Source: three-view drawing plus pictorial views. Frame: mm from the lowest corner of the part. Coordinates: 2 decimals unless noted, no trailing zeros. Write each loop counter-clockwise with the first axis right and the second up, starting at its lowest first coordinate (ties: lowest second). Pieces come first, ordered by that corner, then holes. Notation, with made-up numbers: (-12, 15) -> (13, 15) arc R13 ccw to (13, 22) -> close; hole circle Ø7 at (67, 64.5). An arc over 180 degrees is marked (long way). One line per question, with ' | ' between items. Start each with the question number.
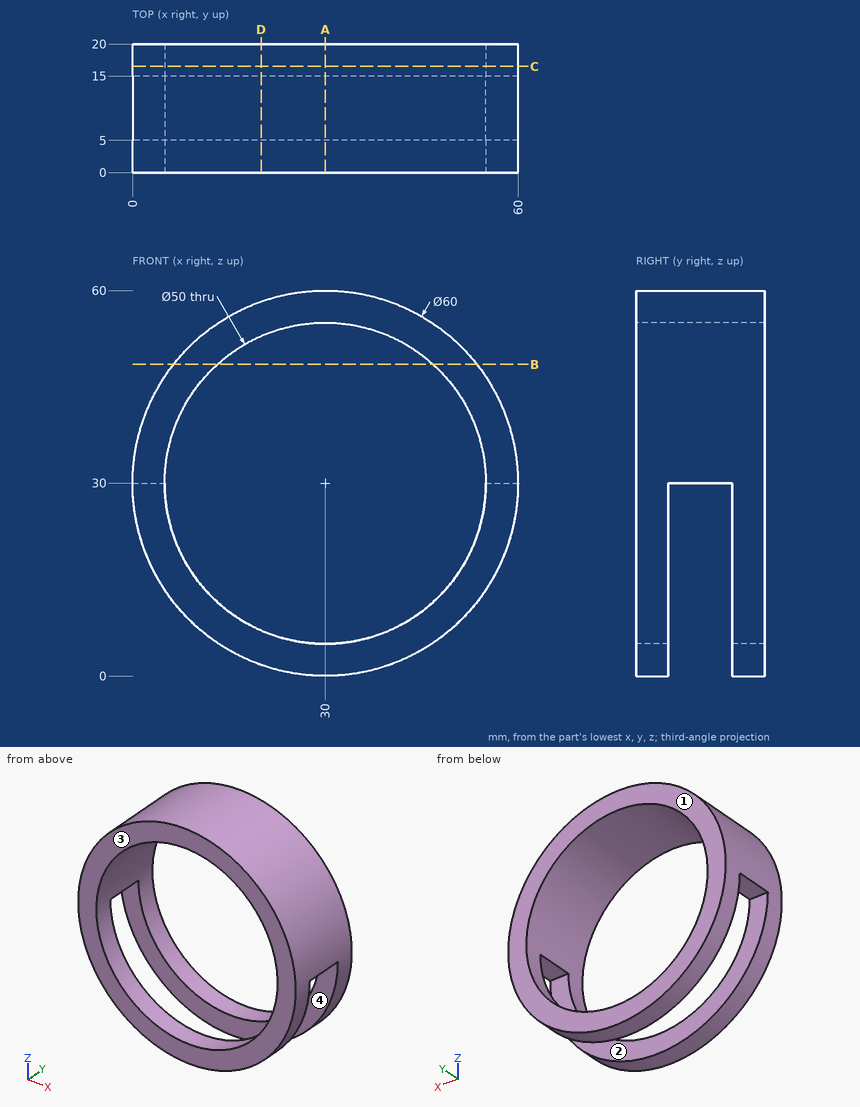
1) Pull-direction query (Y, two-part tool) for the marked faces 1, 2, 3 and 4; classes: released by +Y, released by -Y, zero draft, split by the parting line, or undercut.
2) Section A-A, the plane x = 30. Return loops of the section in (y, z).
3) Ray query, line 1 (Y direction, x = 6, z = 20.5); line 2 (Z direction, x = 44.5, y = 16.5); line 3 (X direction, y = 4, z = 30). Return the intervals inside material, ascending.
4) Section D-D, the plane x = 20. Return loops of the section in (y, z).
5) First-contact query: P1, Ø1.5, axis at y = 12, z = 47, coming from the +X side; P2, Ø1.5, axis at y = 8.5, z = 38, coming from the -X side; P3, Ø4, axis at x = 37, y = 14, coming from the +Z side; P4, Ø9, axis at x = 22.5, z = 14.5, coming from the -Y side. Flat tips, straight axial feed; report the tip coordinate or a pass-through.
6) Section C-C, the plane y = 16.5. Return loops of the section in (x, z), then the cut area to 3 significant figures.
7) Section B-B, the plane z = 48.5. Return loops of the section in (x, y).
Answer block:
1) face 1: released by +Y | face 2: undercut | face 3: released by -Y | face 4: undercut
2) outline: (0, 0) -> (5, 0) -> (5, 5) -> (0, 5) -> close; (0, 55) -> (20, 55) -> (20, 60) -> (0, 60) -> close; (15, 0) -> (20, 0) -> (20, 5) -> (15, 5) -> close
3) line 1: y = 0 to 5, 15 to 20 | line 2: z = 3.74 to 9.63, 50.37 to 56.26 | line 3: x = 0 to 5, 55 to 60
4) outline: (0, 1.72) -> (5, 1.72) -> (5, 7.09) -> (0, 7.09) -> close; (0, 52.91) -> (20, 52.91) -> (20, 58.28) -> (0, 58.28) -> close; (15, 1.72) -> (20, 1.72) -> (20, 7.09) -> (15, 7.09) -> close
5) P1: stops at x = 55.22 | P2: stops at x = 0.89 | P3: stops at z = 59.58 | P4: passes through
6) outline: circle Ø60 at (30, 30); hole circle Ø50 at (30, 30) | area: 864 mm2
7) outline: (6.38, 0) -> (13.18, 0) -> (13.18, 20) -> (6.38, 20) -> close; (46.82, 0) -> (53.62, 0) -> (53.62, 20) -> (46.82, 20) -> close
